Can you work these out from the model? Positions are in its coordinate system, mm. Round coordinates to 2 decimals unless told otherwise and drop trailing zeros. Order: outer loops, then holes, each group sorted by start corner. A loop starts at its lowest first (then second) coordinate and runs counter-clockwise, first axis right, second up. Notation, with made-up numbers: (39.5, 68) -> (70.5, 68) arc R24 ccw to (70.5, 78) -> close; hole circle Ø6 at (88, -26.75). An arc over 180 degrees is marked (long way). Use a Markdown table: item, result. Add a question column.
Q1. I need wall thicknesses on line 1 along Y through (x, z) = (0, -1.25); line 2 along Y through (x, z) = (3, -7.5); line 3 along X through (y, z) = (-0.25, -2.25). Which ranges of each line are inside material? Lowest first, please. Write a range as [from, to].
Q2. If we section it at A-A on x = 0: List the corners of the cut face in (y, z) for me, plus the area to 3 significant figures.
Q3. If we section it at C-C on z = -9: List the corners of the cut face in (x, y) for me.
Q4. If we section it at D-D on y = 3.25: List the corners of the cut face in (x, z) for me, plus the area to 3 significant figures.
Q5. We'd pull the mould along Z, two halves only. Please class faces 1 (the face through (-0.2, -5.4, 12.5)), 2 (the face through (-8.6, -0.9, 7.2)), 3 (the face through (-0.2, -5.4, -12.5)), 4 (the face through (-8.6, -0.9, -4.8)): +Z half, -Z half, draft (parallel to the pull), parting line (faces both ways), or undercut.
Q6. I'm going to push flat-ended pins straight in: pin 1 Ø5 at (x, z) = (4, -6.5) entering from +Y; pin 2 Ø6 at (y, z) = (5.5, 3.5) entering from -X; pin 3 Ø13 at (x, y) = (0, 0) entering from -Z; pin 4 Ø1.5 at (x, z) = (-7, -4.5) entering from -Y. Where does each tip first touch, or does it pass through?
Q7. If we section it at B-B on y = 0: List the corners of the cut face in (x, z) for me.
```python
from build123d import *

# Parameters (mm, degrees)
CROQUIS1_R              = 12.5
SALIENTE_EXTRUIR1_DEPTH = 12.5
CROQUIS2_R              = 5
CORTAR_EXTRUIR1_DEPTH   = 25
CORTAR_EXTRUIR2_REACH   = 14.5
CROQUIS3_R              = 1.5


with BuildPart() as part:
    # Croquis1 → Saliente-Extruir1 (new body, symmetric)
    with BuildSketch(Plane.XY):
        Circle(CROQUIS1_R)
    extrude(amount=SALIENTE_EXTRUIR1_DEPTH, both=True)

    # Croquis2 → Cortar-Extruir1 (cut)
    with BuildSketch(Plane.XY.offset(12.5)):
        Circle(CROQUIS2_R)
    extrude(amount=-CORTAR_EXTRUIR1_DEPTH, mode=Mode.SUBTRACT)

    # Croquis3 → Cortar-Extruir2 (cut, up to next)
    with BuildSketch(Plane(origin=(0, 0, 0), x_dir=(0, 0, -1), z_dir=(1, 0, 0)), mode=Mode.PRIVATE) as cortar_extruir2_sk1:
        with Locations((-6, 0)):
            Circle(CROQUIS3_R)
    cortar_extruir2_tool1 = extrude(cortar_extruir2_sk1.sketch, amount=-CORTAR_EXTRUIR2_REACH, mode=Mode.PRIVATE) & part.part
    add(cortar_extruir2_tool1.solids().sort_by_distance((0, 0, 6))[0], mode=Mode.SUBTRACT)
    # Croquis3 → Cortar-Extruir2 (cut, up to next)
    with BuildSketch(Plane(origin=(0, 0, 0), x_dir=(0, 0, -1), z_dir=(1, 0, 0)), mode=Mode.PRIVATE) as cortar_extruir2_sk2:
        with Locations((6, 0)):
            Circle(CROQUIS3_R)
    cortar_extruir2_tool2 = extrude(cortar_extruir2_sk2.sketch, amount=-CORTAR_EXTRUIR2_REACH, mode=Mode.PRIVATE) & part.part
    add(cortar_extruir2_tool2.solids().sort_by_distance((0, 0, -6))[0], mode=Mode.SUBTRACT)


solid = part.part
```
Answer below:
| question | item | result |
|---|---|---|
| 1 | line 1 | [-12.5, -5], [5, 12.5] |
| 1 | line 2 | [-12.13, -4], [4, 12.13] |
| 1 | line 3 | [-12.5, -4.99], [4.99, 12.5] |
| 2 | outline | (-12.5, -12.5) -> (-5, -12.5) -> (-5, 12.5) -> (-12.5, 12.5) -> close; (5, -12.5) -> (12.5, -12.5) -> (12.5, 12.5) -> (5, 12.5) -> close |
| 2 | area | 375 mm² |
| 3 | outline | circle Ø25 at (0, 0); hole circle Ø10 at (0, 0) |
| 4 | outline | (-12.07, -12.5) -> (-3.8, -12.5) -> (-3.8, 12.5) -> (-12.07, 12.5) -> close; (3.8, -12.5) -> (12.07, -12.5) -> (12.07, 12.5) -> (3.8, 12.5) -> close |
| 4 | area | 414 mm² |
| 5 | face 1 | +Z half |
| 5 | face 2 | undercut |
| 5 | face 3 | -Z half |
| 5 | face 4 | undercut |
| 6 | pin 1 | y = 12.41 |
| 6 | pin 2 | x = -12.25 |
| 6 | pin 3 | z = -12.5 |
| 6 | pin 4 | y = -10.83 |
| 7 | outline | (-12.5, -12.5) -> (-5, -12.5) -> (-5, -7.5) -> (-12.5, -7.5) -> close; (-12.5, -4.5) -> (-5, -4.5) -> (-5, 4.5) -> (-12.5, 4.5) -> close; (-12.5, 7.5) -> (-5, 7.5) -> (-5, 12.5) -> (-12.5, 12.5) -> close; (5, -12.5) -> (12.5, -12.5) -> (12.5, 12.5) -> (5, 12.5) -> close |
